Could you check a few things on this model? Use its own coordinates, in mm. Face numbers are marked on the shaded views. A direction names the side the tool comes from. Coordinates: 2 decimals unless noted, no trailing zeros. Order: outer loops, then holes, each group sorted by start corner. A loop starts at its lowest first (then second) coordinate and runs counter-clockwise, first axis right, second up. Notation, with made-up numbers: (52.5, 34.5) - (92.5, 34.5) arc R15 cw to (92.5, 38.5) - close; hole circle Ø11 at (-16, 3.5). An arc over 180 degrees is marked (long way). One line per item, written item: value.
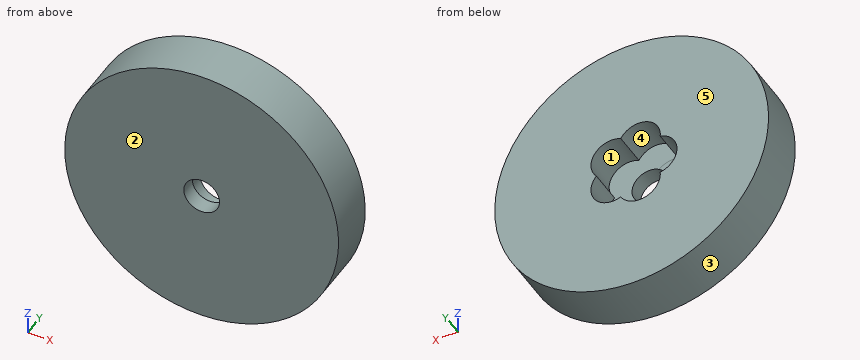
from build123d import *

# Parameters (mm, degrees)
SKETCH1_R           = 57.5
BOSS_EXTRUDE1_DEPTH = 21
SKETCH2_R           = 7.5
CUT_EXTRUDE1_DEPTH  = 84.985117729
SKETCH3_R           = 8.914028006
CUT_EXTRUDE2_DEPTH  = 14.30003
CIRPATTERN1_START   = 6.699969607
CIRPATTERN1_DEPTH   = 14.300030393


# Read off the part's stored shape, not the designer's step: CirPattern1
with BuildPart() as part:
    # Sketch1 → Boss-Extrude1 (new body)
    with BuildSketch(Plane(origin=(0, 0, 0), x_dir=(1, 0, 0), z_dir=(0, 1, 0))):
        with Locations(Location((0, 0, 0), (0, 0, 90))):
            Circle(SKETCH1_R)
    extrude(amount=BOSS_EXTRUDE1_DEPTH)

    # Sketch2 → Cut-Extrude1 (cut, through all)
    with BuildSketch(Plane(origin=(0, 0, 0), x_dir=(1, 0, 0), z_dir=(0, 1, 0))):
        with Locations(Location((0, 0, 0), (0, 0, 90))):
            Circle(SKETCH2_R)
    extrude(amount=CUT_EXTRUDE1_DEPTH, mode=Mode.SUBTRACT)

    # Sketch3 → Cut-Extrude2 (cut)
    with BuildSketch(Plane(origin=(0, 21, 0), x_dir=(1, 0, 0), z_dir=(0, 1, 0))):
        with Locations((-10.109024176, 0)):
            Circle(SKETCH3_R)
    extrude(amount=-CUT_EXTRUDE2_DEPTH, mode=Mode.SUBTRACT)

    # CirPattern1 outline → CirPattern1 (cut)
    with BuildSketch(Plane(origin=(0, 0, 0), x_dir=(1, 0, 0), z_dir=(0, 1, 0)).offset(CIRPATTERN1_START)):
        with BuildLine():
            ThreePointArc((-3.906533071, -6.402265175), (-7.659774999, -8.570943574), (-11.992194257, -8.712839132))
            ThreePointArc((-11.992194257, -8.712839132), (-5.878446409, -18.091997737), (4.580610606, -14.097669853))
            ThreePointArc((4.580610606, -14.097669853), (15.3899725, -11.181469526), (14.823167301, 0))
            ThreePointArc((14.823167301, 0), (15.3899725, 11.181469526), (4.580610606, 14.097669853))
            ThreePointArc((4.580610606, 14.097669853), (-5.878446409, 18.091997737), (-11.992194257, 8.712839132))
            ThreePointArc((-11.992194257, 8.712839132), (-7.659774999, 8.570943574), (-3.906533071, 6.402265175))
            ThreePointArc((-3.906533071, 6.402265175), (7.5, 0), (-3.906533071, -6.402265175))
        make_face()
    extrude(amount=CIRPATTERN1_DEPTH, mode=Mode.SUBTRACT)


solid = part.part
Item 1: I want a section at C-C on y = 2.75. Please give me the cut outline in (x, z), then the cut area to 3 significant figures.
Conclusion:
outline: circle Ø115 at (0, 0); hole circle Ø15 at (0, 0)
area: 10,200 mm²
Item 2: For the marked faces 4 and 5, which set-ups out of +Z, -Z, +X, -X, +Y, -Y let a thin tool reach every point of the face, with its end or its side?
Conclusion:
face 4: +Y
face 5: +Z, -Z, +X, -X, +Y
Item 3: If I drill on probe 1 along X at (y, z) = (3.5, 0); probe 2 along X at (y, z) = (13, -3.5); probe 3 along X at (y, z) = (3.5, 20), over which ranges is the centre line in solid material (lowest first)?
Conclusion:
probe 1: -57.5 to -7.5, 7.5 to 57.5
probe 2: -57.39 to -18.31, 16.75 to 57.39
probe 3: -53.91 to 53.91
Item 4: I want a section at A-A on x = 0. Please give me the cut outline in (y, z), then the cut area to 3 significant figures.
Conclusion:
outline: (0, -57.5) - (21, -57.5) - (21, -17.96) - (6.7, -17.96) - (6.7, -7.5) - (0, -7.5) - close; (0, 7.5) - (6.7, 7.5) - (6.7, 17.96) - (21, 17.96) - (21, 57.5) - (0, 57.5) - close
area: 1,800 mm²
Item 5: I want a section at B-B on z = 1.5. Please give me the cut outline in (x, y), then the cut area to 3 significant figures.
Conclusion:
outline: (-57.48, 0) - (-7.35, 0) - (-7.35, 6.7) - (-18.9, 6.7) - (-18.9, 21) - (-57.48, 21) - close; (7.35, 0) - (57.48, 0) - (57.48, 21) - (15.91, 21) - (15.91, 6.7) - (7.35, 6.7) - close
area: 1,820 mm²
Item 6: I'm going to push flat-ended pins straight in: pin 1 Ø12 at (x, y) = (27, 4) entering from +Z; pin 2 Ø13.5 at (x, z) = (0, 0) entering from +Y; pin 3 Ø14.5 at (x, z) = (2.5, 1.5) entering from +Y; pin 4 Ø8 at (y, z) = (16.5, 29) entering from +X. Where does each tip first touch, or does it pass through?
Conclusion:
pin 1: z = 53.53
pin 2: through
pin 3: y = 6.7
pin 4: x = 51.78
Item 7: I want a section at D-D on x = 11.5. Please give me the cut outline in (y, z).
Conclusion:
outline: (0, -56.34) - (21, -56.34) - (21, -14.21) - (6.7, -14.21) - (6.7, 14.21) - (21, 14.21) - (21, 56.34) - (0, 56.34) - close
Item 8: Thinking about a two-plate mould opening in Z: for the marked faces 1, 2 and 3, which applies, pulls with the +Z half, pulls with the -Z half, needs draft (parallel to the pull), parting line crosses it, or undercut?
Conclusion:
face 1: undercut
face 2: needs draft
face 3: parting line crosses it
